from build123d import *

# Parameters (mm, degrees)
F1_DEPTH = 603.25
F3_DEPTH = 38.101
F4_R     = 6.35
F5_DEPTH = 1.5875
F6_R     = 1.5875
F7_DEPTH = 3.175


with BuildPart() as f1:
    # F0 (on Front) → F1 (new body, symmetric)
    with BuildSketch(Plane.XZ):
        Polygon((-19.05, -31.75), (19.05, -31.75), (19.05, 31.75), (11.1125, 31.75), (11.1125, 21.59), (7.9375, 21.59), (7.9375, 31.75), (-7.9375, 31.75), (-7.9375, 21.59), (-11.1125, 21.59), (-11.1125, 31.75), (-19.05, 31.75), align=None)
    extrude(amount=F1_DEPTH, both=True)

    # F2 (on face) → F3 (cut, through all)
    with BuildSketch(Plane(origin=(-19.05, 0, 0), x_dir=(0, -1, 0), z_dir=(-1, 0, 0))):
        Polygon((539.75, 31.75), (603.25, -31.75), (603.25, 31.75), align=None)
        Polygon((-603.25, 31.75), (-603.25, -31.75), (-539.75, 31.75), align=None)
    extrude(amount=-F3_DEPTH, mode=Mode.SUBTRACT)

    # F4 (on face) → F5 (cut)
    with BuildSketch(Plane(origin=(-19.05, 0, 0), x_dir=(0, -1, 0), z_dir=(-1, 0, 0))):
        with Locations((539.75, -12.7)):
            Circle(F4_R)
        with Locations((-539.75, -12.7)):
            Circle(F4_R)
    extrude(amount=-F5_DEPTH, mode=Mode.SUBTRACT)

    # F6 (on face) → F7 (cut)
    with BuildSketch(Plane(origin=(-19.05, 0, 0), x_dir=(0, -1, 0), z_dir=(-1, 0, 0))):
        with Locations((269.875, -12.7)):
            Circle(F6_R)
        with Locations((-269.875, -12.7)):
            Circle(F6_R)
    extrude(amount=-F7_DEPTH, mode=Mode.SUBTRACT)


solid = f1.part
Can you work these out from the model? Positions are in its coordinate system, mm. Give positions to 0.01 mm unless a question says otherwise; leave off trailing zeros. Write each loop counter-clockwise with the first axis right and the second up, starting at its lowest first coordinate (ties: lowest second). Pieces come first, ordered by that corner, then holes. Notation, with made-up numbers: M 57,-22.5 L 98,-22.5 A21 ccw 98,-12.5 Z; hole C 17.25,-2 d4. An arc over 180 degrees is marked long. Answer in a Markdown table with one row per item. Add a question column.
Item 1: Imagine slicing it at B-B, the plane z = 10.5. Write out the boundary of the cut face in (x, y).
Item 2: Please list where these lines run through material, in increasing order: L1, parallel to X at y = -81, z = 22; L2, parallel to Y at x = -16, z = -12; L3, parallel to Z at x = -10, y = -426.5.
Item 3: For pin 1 Ø7.5 at (y, z) = (539.75, -12.7) entering from -X; pin 2 Ø1.6 at (x, y) = (9.5, -48.5) entering from +Z; pin 3 Ø1 at (x, z) = (8, 14) entering from -Y; pin 4 Ø2.5 at (y, z) = (-269.5, -12.5) entering from -X, each with a flat end and sliding along its axis, tell me the tip position at first contact or that it passes through.
Item 4: Imagine slicing it at A-A, the plane y = -511.5. Write out the boundary of the cut face in (x, z), plus the area to 3 significant figures.
Evaluation:
| question | item | result |
|---|---|---|
| 1 | outline | M -19.05,-561 L 19.05,-561 L 19.05,561 L -19.05,561 Z |
| 2 | L1 | x = -19.05 to -11.11, -7.94 to 7.94, 11.11 to 19.05 |
| 2 | L2 | y = -583.5 to -271.3, -268.45 to 268.45, 271.3 to 583.5 |
| 2 | L3 | z = -31.75 to 21.59 |
| 3 | pin 1 | stops at x = -17.46 |
| 3 | pin 2 | stops at z = 21.59 |
| 3 | pin 3 | stops at y = -558 |
| 3 | pin 4 | stops at x = -19.05 |
| 4 | outline | M -19.05,-31.75 L 19.05,-31.75 L 19.05,31.75 L 11.11,31.75 L 11.11,21.59 L 7.94,21.59 L 7.94,31.75 L -7.94,31.75 L -7.94,21.59 L -11.11,21.59 L -11.11,31.75 L -19.05,31.75 Z |
| 4 | area | 2,350 mm² |
